Here's how the part is built. I have some questions about the finished solid (model axes, mm). Face numbers are marked on the shaded views. A direction names the side the tool comes from. Round coordinates to 2 decimals unless told otherwise and drop trailing zeros. Write each loop counter-clockwise with the first axis right and the second up, starting at its lowest first coordinate (ties: lowest second). Pieces come first, ordered by that corner, then holes. Notation, with made-up numbers: (-2, 34.25) -> (42, 34.25) arc R16 ccw to (42, 55.25) -> close; hole circle Ø7 at (84, 1.25). An arc over 180 degrees is marked (long way). Answer as CSV lines item,"result".
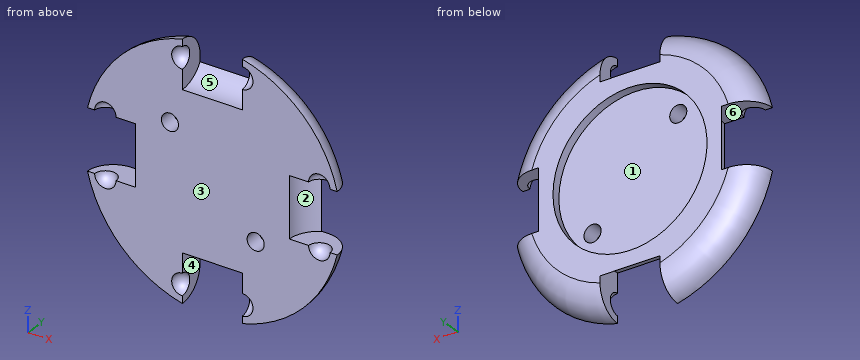
Autodesk Inventor part; units mm, degrees
ref_plane "YZ Plane" through (0, 0, 0) normal (1, 0, 0) x (0, 1, 0)
ref_plane "XZ Plane" through (0, 0, 0) normal (0, 1, 0) x (-1, 0, 0)
ref_plane "XY Plane" through (0, 0, 0) normal (0, 0, 1) x (1, 0, 0)
sketch "Sketch1" plane through (0, 0, 0) normal (0, 1, 0) x (-1, 0, 0)
  circle A0 centre (0, 0) radius 30
  dimension "d0" = 60
extrude "Extrusion1" add sketch "Sketch1" along normal blind 6
fillet "Fillet1" radius 6 1 edges at (30, 6, 0)
sketch "Sketch2" plane through (0, 0, 0) normal (0, -1, 0) x (1, 0, 0)
  line L0 (-7, -25) -> (7, -25)
  line L1 (7, -25) -> (7, -18)
  line L2 (7, -18) -> (-7, -18)
  line L3 (-7, -18) -> (-7, -25)
  line L4 (-7, -25) -> (7, -18) construction
  line L5 (7, -25) -> (-7, -18) construction
  arc A0 (-4.5, -25) -> (-9.5, -25) centre (-7, -25) ccw
  arc A1 (9.5, -25) -> (4.5, -25) centre (7, -25) ccw
  line L6 (-9.5, -25) -> (9.5, -25)
  point P0 (0, 0)
  point P1 (0, -21.5)
  dimension "d4" = 14
  dimension "d5" = 7
  dimension "d6" = 18
  dimension "d7" = 5
  dimension "d8" = 5
revolve "Revolution1" cut sketch "Sketch2" angle 360 about axis through (-7, 0, -25) along (1, 0, 0)
pattern_circular "Circular Pattern1" count 4 over 360 about axis through (0, -10, 0) along (0, 1, 0) of "Revolution1"
sketch "Sketch3" plane through (0, 6, 0) normal (0, 1, 0) x (1, 0, 0)
  circle A0 centre (0, 0) radius 18
  dimension "d13" = 36
extrude "Extrusion2" cut sketch "Sketch3" against normal blind 2
sketch "Sketch4" plane through (0, 4, 0) normal (0, 1, 0) x (1, 0, 0)
  line L0 (0, 0) -> (0, -8.2559)
  line L1 (0, 0) -> (-9.8995, -9.8995)
  line L2 (0, 0) -> (9.8995, 9.8995)
  point P0 (10.1305, 10.1305)
  dimension "d16" = 45
  dimension "d17" = 14
  dimension "d18" = 14
hole "Hole1" at (-9.8995, 4, 9.8995) at (10.1305, 4, -10.1305) direction (0, -1, 0) diameter 4 end through all
properties part number "omni_wheel_cover_in"
Item 1: For the marked faces 4, 5 and 6, which set-ups out of +Z, -Z, +X, -X, +Y, -Y let a thin tool reach every point of the face, with its end or its side?
Results found:
face 4,"-Z, -Y"
face 5,"+Z, -Y"
face 6,"-X, -Y"
Item 2: Will these pins go through, and if not, where does the flat tip stop? pin 1 (3 mm diameter, centred on x = 24, y = 4, fed in from +Z); pin 2 (3 mm diameter, centred on y = 4, z = -2.5, fed in from +X); pin 3 (5 mm diameter, centred on x = 10.13, z = -10.13, fed in from +Y).
Results found:
pin 1,"stops at z = 18.14"
pin 2,"stops at x = 20.67"
pin 3,"stops at y = 4"
Item 3: Suppose I cut it at B-B, the plane y = 0.75. State how many separate pieces and enclosed holes the cut face has, then the cut area to 3 significant figures.
Results found:
separate pieces,"1"
enclosed holes,"2"
area,"2,070 mm²"
Item 4: If we mould it in two halves opening along X, with no side actions, what happens to the marked faces 1, 2 and 3? For each: pulls with the +X half, pulls with the -X half, needs draft (parallel to the pull), parting line crosses it, or undercut.
Results found:
face 1,"undercut"
face 2,"pulls with the +X half"
face 3,"needs draft"
Item 5: I need wall thicknesses on L1, parallel to Y at x = 14, z = 11; L2, parallel to Z at x = 3, y = 5; L3, parallel to Z at x = -4, y = 4.75. Which ranges of each line are inside material? Lowest first, please.
Results found:
L1,"y = 0 to 4"
L2,"z = -20.1 to -17.75, 17.75 to 20.1"
L3,"z = -19.86 to -17.55, 17.55 to 19.86"
Item 6: Suppose I cut it at D-D, the plane y = 5. List the corners of the cut face in (x, z) for me, then the cut area to 3 significant figures.
Results found:
outline,"(-26.4, -7) arc R27.32 ccw to (-7, -26.4) -> (-7, -20.1) -> (7, -20.1) -> (7, -26.4) arc R27.32 ccw to (26.4, -7) -> (20.1, -7) -> (20.1, 7) -> (26.4, 7) arc R27.32 ccw to (7, 26.4) -> (7, 20.1) -> (-7, 20.1) -> (-7, 26.4) arc R27.32 ccw to (-26.4, 7) -> (-20.1, 7) -> (-20.1, -7) -> close; hole circle Ø36 at (0, 0)"
area,"939 mm²"
Item 7: Suppose I cut it at A-A, the plane x = 0. List the corners of the cut face in (y, z) for me.
Results found:
outline,"(0, -18) arc R7 cw to (6, -21.39) -> (6, -18) -> (4, -18) -> (4, 18) -> (6, 18) -> (6, 21.39) arc R7 cw to (0, 18) -> close"
Item 8: Suppose I cut it at C-C, the plane z = 0. List the corners of the cut face in (x, y) for me.
Results found:
outline,"(-21.39, 6) arc R7 cw to (-18, 0) -> (18, 0) arc R7 cw to (21.39, 6) -> (18, 6) -> (18, 4) -> (-18, 4) -> (-18, 6) -> close"
